For this review, take the finished solid that the model builds, in its own axes (mm). Round coordinates to 2 decimals unless told otherwise and drop trailing zeros. Order: outer loops, then holes, each group sorted by start corner. A loop starts at its lowest first (then second) coordinate and runs counter-clockwise, first axis right, second up. Notation, with made-up numbers: M 24.25,2 L 48.25,2 A18 cw 48.25,25 Z; hole C 67,-13.75 d9. An arc over 180 degrees is marked long. Answer in a Markdown table with one row per item. Add a question column.
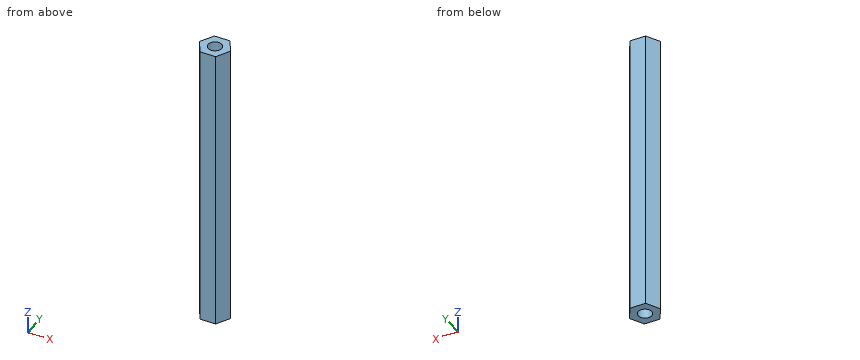
```python
from build123d import *

# Parameters (mm, degrees)
F_70MM_DEPTH           = 65
SKETCH_M3_R            = 1.51
CUT_EXTRUDE_M3_DEPTH   = 8
CUT_EXTRUDE_START      = -8
SKETCH_M3_2_R          = 1.51
CUT_EXTRUDE_M3_2_DEPTH = 8


with BuildPart() as part:
    # Sketch 185 → 隔柱高度_70mm (new body)
    with BuildSketch(Plane.XY):
        Polygon((3.464101615, 0), (1.732050808, 3), (-1.732050808, 3), (-3.464101615, 0), (-1.732050808, -3), (1.732050808, -3), align=None)
    extrude(amount=F_70MM_DEPTH)

    # Sketch M3 → Cut-Extrude M3 (cut)
    with BuildSketch(Plane(origin=(0, 0, 0), x_dir=(-1, 0, 0), z_dir=(0, 0, -1))):
        Circle(SKETCH_M3_R)
    extrude(amount=-CUT_EXTRUDE_M3_DEPTH, mode=Mode.SUBTRACT)

    # Sketch M3 2 → Cut-Extrude M3 2 (cut)
    with BuildSketch(Plane.XY.offset(65).offset(CUT_EXTRUDE_START)):
        with Locations(Location((0, 0, 0), (0, 0, 180))):
            Circle(SKETCH_M3_2_R)
    extrude(amount=CUT_EXTRUDE_M3_2_DEPTH, mode=Mode.SUBTRACT)


solid = part.part
```
1. Clearance check with flat-ended pins moving along their axes: pin 1 Ø2.5 at (x, y) = (0, -0.5) entering from +Z; pin 2 Ø1 at (y, z) = (-1.5, 42.5) entering from +X; pin 3 Ø0.9 at (x, y) = (0.5, -0.5) entering from -Z. State where each tip first meets the part, or that it passes through.
2. Consider section A-A on x = 0. Write out the cut boundary in (y, z), plus the area to 3 significant figures.
3. Consider section C-C on y = -0.75. Write out the cut boundary in (x, z), plus the area to 3 significant figures.
4. To check wall thickness, follow probe 1 along Y at (x, z) = (0, 62.75); probe 2 along Z at (x, y) = (-0.75, 0.25); probe 3 along X at (y, z) = (-1.25, 61). State the ranges of each line that lie inside material, in increasing order. Write a range as [from, to].
5. Consider section B-B on z = 40.5. Write out the cut boundary in (x, y), plus the area to 3 significant figures.
6. Consider section D-D on x = 2.75. Write out the cut boundary in (y, z), plus the area to 3 significant figures.
Solved:
| question | item | result |
|---|---|---|
| 1 | pin 1 | stops at z = 65 |
| 1 | pin 2 | stops at x = 2.89 |
| 1 | pin 3 | stops at z = 8 |
| 2 | outline | M -3,0 L -1.51,0 L -1.51,8 L 1.51,8 L 1.51,0 L 3,0 L 3,65 L 1.51,65 L 1.51,57 L -1.51,57 L -1.51,65 L -3,65 Z |
| 2 | area | 342 mm^2 |
| 3 | outline | M -3.03,0 L -1.31,0 L -1.31,8 L 1.31,8 L 1.31,0 L 3.03,0 L 3.03,65 L 1.31,65 L 1.31,57 L -1.31,57 L -1.31,65 L -3.03,65 Z |
| 3 | area | 352 mm^2 |
| 4 | probe 1 | y = [-3, -1.51], [1.51, 3] |
| 4 | probe 2 | z = [8, 57] |
| 4 | probe 3 | x = [-2.74, -0.85], [0.85, 2.74] |
| 5 | outline | M -3.46,0 L -1.73,-3 L 1.73,-3 L 3.46,0 L 1.73,3 L -1.73,3 Z |
| 5 | area | 31.2 mm^2 |
| 6 | outline | M -1.24,0 L 1.24,0 L 1.24,65 L -1.24,65 Z |
| 6 | area | 161 mm^2 |
